```python
from build123d import *

# Parameters (mm, degrees)
SKETCH_1_R          = 45
EXTRUDE_1_DEPTH     = 5
SKETCH_2_W          = 60
SKETCH_2_H          = 60
EXTRUDE_2_DEPTH     = 5
CUT_EXTRUDE_1_DEPTH = 10
CUT_EXTRUDE_START   = -50
CUT_EXTRUDE_2_DEPTH = 10
CUT_EXTRUDE_3_DEPTH = 17
CUT_EXTRUDE_START_2 = -43
CUT_EXTRUDE_4_DEPTH = 17
CUT_EXTRUDE_5_REACH = 89.607
CHAMFER_1_SIZE      = 5
SKETCH_6_R          = 17.5
CUT_EXTRUDE_6_DEPTH = 3
SKETCH_7_R          = 15
CUT_EXTRUDE_7_DEPTH = 65.02343321
SKETCH_8_R          = 45
CUT_EXTRUDE_9_DEPTH = 10


with BuildPart() as part:
    # 草图1 → 凸台-拉伸1 (new body)
    with BuildSketch(Plane.XY):
        Circle(SKETCH_1_R)
    extrude(amount=-EXTRUDE_1_DEPTH)

    # 草图2 → 凸台-拉伸2 (add)
    with BuildSketch(Plane.XY):
        Rectangle(SKETCH_2_W, SKETCH_2_H)
    extrude(amount=EXTRUDE_2_DEPTH)

    # 草图3 → 切除-拉伸1 (cut)
    with BuildSketch(Plane.XZ.offset(30)):
        with BuildLine():
            Line((-1.5, 5), (1.5, 5))
            Line((1.5, 5), (1.5, 4.322875656))
            ThreePointArc((1.5, 4.322875656), (1.780042303, 3.911838473), (1.95, 3.444409721))
            Line((1.95, 3.444409721), (1.95, 2.2))
            Line((1.95, 2.2), (-1.95, 2.2))
            Line((-1.95, 2.2), (-1.95, 3.444409721))
            ThreePointArc((-1.95, 3.444409721), (-1.780042303, 3.911838473), (-1.5, 4.322875656))
            Line((-1.5, 4.322875656), (-1.5, 5))
        make_face()
        with BuildLine():
            Line((6, 5), (6, 4.322875656))
            ThreePointArc((6, 4.322875656), (5.719957697, 3.911838473), (5.55, 3.444409721))
            Line((5.55, 3.444409721), (5.55, 2.2))
            Line((5.55, 2.2), (9.45, 2.2))
            Line((9.45, 2.2), (9.45, 3.444409721))
            ThreePointArc((9.45, 3.444409721), (9.280042303, 3.911838473), (9, 4.322875656))
            Line((9, 4.322875656), (9, 5))
            Line((9, 5), (6, 5))
        make_face()
        with BuildLine():
            Line((-9, 5), (-9, 4.322875656))
            ThreePointArc((-9, 4.322875656), (-9.280042303, 3.911838473), (-9.45, 3.444409721))
            Line((-9.45, 3.444409721), (-9.45, 2.2))
            Line((-9.45, 2.2), (-5.55, 2.2))
            Line((-5.55, 2.2), (-5.55, 3.444409721))
            ThreePointArc((-5.55, 3.444409721), (-5.719957697, 3.911838473), (-6, 4.322875656))
            Line((-6, 4.322875656), (-6, 5))
            Line((-6, 5), (-9, 5))
        make_face()
    extrude(amount=-CUT_EXTRUDE_1_DEPTH, mode=Mode.SUBTRACT)

    # 草图3<2> → 切除-拉伸2 (cut)
    with BuildSketch(Plane.XZ.offset(30).offset(CUT_EXTRUDE_START)):
        with BuildLine():
            Line((-1.5, 5), (1.5, 5))
            Line((1.5, 5), (1.5, 4.322875656))
            ThreePointArc((1.5, 4.322875656), (1.780042303, 3.911838473), (1.95, 3.444409721))
            Line((1.95, 3.444409721), (1.95, 2.2))
            Line((1.95, 2.2), (-1.95, 2.2))
            Line((-1.95, 2.2), (-1.95, 3.444409721))
            ThreePointArc((-1.95, 3.444409721), (-1.780042303, 3.911838473), (-1.5, 4.322875656))
            Line((-1.5, 4.322875656), (-1.5, 5))
        make_face()
        with BuildLine():
            Line((6, 5), (6, 4.322875656))
            ThreePointArc((6, 4.322875656), (5.719957697, 3.911838473), (5.55, 3.444409721))
            Line((5.55, 3.444409721), (5.55, 2.2))
            Line((5.55, 2.2), (9.45, 2.2))
            Line((9.45, 2.2), (9.45, 3.444409721))
            ThreePointArc((9.45, 3.444409721), (9.280042303, 3.911838473), (9, 4.322875656))
            Line((9, 4.322875656), (9, 5))
            Line((9, 5), (6, 5))
        make_face()
        with BuildLine():
            Line((-9, 5), (-9, 4.322875656))
            ThreePointArc((-9, 4.322875656), (-9.280042303, 3.911838473), (-9.45, 3.444409721))
            Line((-9.45, 3.444409721), (-9.45, 2.2))
            Line((-9.45, 2.2), (-5.55, 2.2))
            Line((-5.55, 2.2), (-5.55, 3.444409721))
            ThreePointArc((-5.55, 3.444409721), (-5.719957697, 3.911838473), (-6, 4.322875656))
            Line((-6, 4.322875656), (-6, 5))
            Line((-6, 5), (-9, 5))
        make_face()
    extrude(amount=-CUT_EXTRUDE_2_DEPTH, mode=Mode.SUBTRACT)

    # 草图4 → 切除-拉伸3 (cut)
    with BuildSketch(Plane.XZ.offset(30)):
        with BuildLine():
            Line((-16.5, 5), (-13.5, 5))
            Line((-13.5, 5), (-13.5, 4.322875656))
            ThreePointArc((-13.5, 4.322875656), (-13.219957697, 3.911838473), (-13.05, 3.444409721))
            Line((-13.05, 3.444409721), (-13.05, 2.2))
            Line((-13.05, 2.2), (-16.95, 2.2))
            Line((-16.95, 2.2), (-16.95, 3.444409721))
            ThreePointArc((-16.95, 3.444409721), (-16.780042303, 3.911838473), (-16.5, 4.322875656))
            Line((-16.5, 4.322875656), (-16.5, 5))
        make_face()
        with BuildLine():
            Line((13.5, 5), (16.5, 5))
            Line((16.5, 5), (16.5, 4.322875656))
            ThreePointArc((16.5, 4.322875656), (16.780042303, 3.911838473), (16.95, 3.444409721))
            Line((16.95, 3.444409721), (16.95, 2.2))
            Line((16.95, 2.2), (13.05, 2.2))
            Line((13.05, 2.2), (13.05, 3.444409721))
            ThreePointArc((13.05, 3.444409721), (13.219957697, 3.911838473), (13.5, 4.322875656))
            Line((13.5, 4.322875656), (13.5, 5))
        make_face()
    extrude(amount=-CUT_EXTRUDE_3_DEPTH, mode=Mode.SUBTRACT)

    # 草图4<2> → 切除-拉伸4 (cut)
    with BuildSketch(Plane.XZ.offset(30).offset(CUT_EXTRUDE_START_2)):
        with BuildLine():
            Line((-16.5, 5), (-13.5, 5))
            Line((-13.5, 5), (-13.5, 4.322875656))
            ThreePointArc((-13.5, 4.322875656), (-13.219957697, 3.911838473), (-13.05, 3.444409721))
            Line((-13.05, 3.444409721), (-13.05, 2.2))
            Line((-13.05, 2.2), (-16.95, 2.2))
            Line((-16.95, 2.2), (-16.95, 3.444409721))
            ThreePointArc((-16.95, 3.444409721), (-16.780042303, 3.911838473), (-16.5, 4.322875656))
            Line((-16.5, 4.322875656), (-16.5, 5))
        make_face()
        with BuildLine():
            Line((13.5, 5), (16.5, 5))
            Line((16.5, 5), (16.5, 4.322875656))
            ThreePointArc((16.5, 4.322875656), (16.780042303, 3.911838473), (16.95, 3.444409721))
            Line((16.95, 3.444409721), (16.95, 2.2))
            Line((16.95, 2.2), (13.05, 2.2))
            Line((13.05, 2.2), (13.05, 3.444409721))
            ThreePointArc((13.05, 3.444409721), (13.219957697, 3.911838473), (13.5, 4.322875656))
            Line((13.5, 4.322875656), (13.5, 5))
        make_face()
    extrude(amount=-CUT_EXTRUDE_4_DEPTH, mode=Mode.SUBTRACT)

    # 草图5 → 切除-拉伸5 (cut, up to next)
    with BuildSketch(Plane.XZ.offset(30), mode=Mode.PRIVATE) as cut_extrude_5_sk1:
        with BuildLine():
            Line((-21, 5), (-21, 4.322875656))
            ThreePointArc((-21, 4.322875656), (-20.719957697, 3.911838473), (-20.55, 3.444409721))
            Line((-20.55, 3.444409721), (-20.55, 2.2))
            Line((-20.55, 2.2), (-24.45, 2.2))
            Line((-24.45, 2.2), (-24.45, 3.444409721))
            ThreePointArc((-24.45, 3.444409721), (-24.280042303, 3.911838473), (-24, 4.322875656))
            Line((-24, 4.322875656), (-24, 5))
            Line((-24, 5), (-21, 5))
        make_face()
    cut_extrude_5_tool1 = extrude(cut_extrude_5_sk1.sketch, amount=-CUT_EXTRUDE_5_REACH, mode=Mode.PRIVATE) & part.part
    # 草图5 → 切除-拉伸5 (cut, up to next)
    with BuildSketch(Plane.XZ.offset(30), mode=Mode.PRIVATE) as cut_extrude_5_sk2:
        with BuildLine():
            Line((24, 5), (24, 4.322875656))
            ThreePointArc((24, 4.322875656), (24.280042303, 3.911838473), (24.45, 3.444409721))
            Line((24.45, 3.444409721), (24.45, 2.2))
            Line((24.45, 2.2), (20.55, 2.2))
            Line((20.55, 2.2), (20.55, 3.444409721))
            ThreePointArc((20.55, 3.444409721), (20.719957697, 3.911838473), (21, 4.322875656))
            Line((21, 4.322875656), (21, 5))
            Line((21, 5), (24, 5))
        make_face()
    cut_extrude_5_tool2 = extrude(cut_extrude_5_sk2.sketch, amount=-CUT_EXTRUDE_5_REACH, mode=Mode.PRIVATE) & part.part
    add(cut_extrude_5_tool1.solids().sort_by_distance((-22.5, -30, 3.520698))[0], mode=Mode.SUBTRACT)
    add(cut_extrude_5_tool2.solids().sort_by_distance((22.5, -30, 3.520698))[0], mode=Mode.SUBTRACT)

    # 倒角1
    chamfer_1_edges = [part.edges().sort_by_distance(p)[0] for p in [
        (-30, 30, 2.5),
        (-30, -30, 2.5),
        (30, -30, 2.5),
        (30, 30, 2.5),
    ]]
    chamfer(chamfer_1_edges, length=CHAMFER_1_SIZE)

    # 草图6 → 切除-拉伸6 (cut)
    with BuildSketch(Plane.XY.offset(5)):
        Circle(SKETCH_6_R)
    extrude(amount=-CUT_EXTRUDE_6_DEPTH, mode=Mode.SUBTRACT)

    # 草图7 → 切除-拉伸7 (cut, through all)
    with BuildSketch(Plane.XY.offset(2)):
        Circle(SKETCH_7_R)
    extrude(amount=-CUT_EXTRUDE_7_DEPTH, mode=Mode.SUBTRACT)

    # 草图8 → 切除-拉伸9 (cut)
    with BuildSketch(Plane.XY):
        Circle(SKETCH_8_R)
    extrude(amount=-CUT_EXTRUDE_9_DEPTH, mode=Mode.SUBTRACT)


solid = part.part
```
For this review, take the finished solid that the model builds, in its own axes (mm). A direction names the side the tool comes from. Round coordinates to 2 decimals unless told otherwise and drop trailing zeros. Write each loop counter-clockwise with the first axis right and the second up, starting at its lowest first coordinate (ties: lowest second). Pieces come first, ordered by that corner, then holes. Notation, with made-up numbers: (74, 49.5) - (133, 49.5) arc R21 cw to (133, 57.5) - close; hole circle Ø8 at (74.25, -35.75). An arc over 180 degrees is marked (long way). Answer as CSV lines item,"result". Start each with the question number.
(1) Add section D-D, the plane x = 11. State the section outline as (y, z) points, plus the area to 3 significant figures.
(2) Add section B-B, the plane y = 0. State the section outline as (x, z) points, plus the area to 3 significant figures.
(3) Machinability: for faces 1 (the cylindrical face through (-13.887, -10.648, 3.521)), 2 (the flat face through (0, -25, 2.2)), 3 (the flat face through (23, 0, 2.2)), 4 (the flat face through (-8, 20, 4)), which of the approach directions +Z, -Z, +X, -X, +Y, -Y give a long, thin tool a straight path to every point of the face, cutting with its end or side? Answer none if there is none.
(4) Add section C-C, the plane z = 1.05. State the section outline as (x, y) points.
(5) Mouldability with a two-part tool opening along Y and no side actions: class faces 5 (the flat face through (15, -22, 2.2)), 6 (the cylindrical face through (-14.985, 0.66, 1.014)), 7 (the flat face through (-8, -20, 4)) as +Y half, -Y half, draft (parallel to the pull), parting line (faces both ways), or undercut.
(6) For line 1 (Y direction, x = 0, z = 1.15); line 2 (Y direction, x = 0, z = 3.75); line 3 (X direction, y = -5, z = 1.4), list the stretches that pass through material, from the lowest coordinate up.
(7) For pin 1 (0.8 mm diameter, centred on x = 14.5, z = 3.5, fed in from +Y); pin 2 (0.8 mm diameter, centred on x = -8, z = 4, fed in from -Y); pin 3 (0.8 mm diameter, centred on x = 15.5, z = 4, fed in from -Y), all flat-tipped, find the tip position at first contact; note any pin that passes through.
(8) Add section A-A, the plane x = 0. State the section outline as (y, z) points, plus the area to 3 significant figures.
From the geometry:
1,outline,"(-30, 0) - (-10.2, 0) - (-10.2, 2) - (-13.61, 2) - (-13.61, 5) - (-30, 5) - close; (10.2, 0) - (30, 0) - (30, 5) - (13.61, 5) - (13.61, 2) - (10.2, 2) - close"
1,area,"178 mm²"
2,outline,"(-30, 0) - (-15, 0) - (-15, 2) - (-17.5, 2) - (-17.5, 5) - (-21, 5) - (-21, 4.32) arc R2 cw to (-20.55, 3.44) - (-20.55, 2.2) - (-24.45, 2.2) - (-24.45, 3.44) arc R2 cw to (-24, 4.32) - (-24, 5) - (-30, 5) - close; (15, 0) - (30, 0) - (30, 5) - (24, 5) - (24, 4.32) arc R2 cw to (24.45, 3.44) - (24.45, 2.2) - (20.55, 2.2) - (20.55, 3.44) arc R2 cw to (21, 4.32) - (21, 5) - (17.5, 5) - (17.5, 2) - (15, 2) - close"
2,area,"115 mm²"
3,face 1,"+Z"
3,face 2,"-Y"
3,face 3,"+Y, -Y"
3,face 4,"+Y"
4,outline,"(-30, -25) - (-25, -30) - (25, -30) - (30, -25) - (30, 25) - (25, 30) - (-25, 30) - (-30, 25) - close; hole circle Ø30 at (0, 0)"
5,face 5,"draft"
5,face 6,"undercut"
5,face 7,"-Y half"
6,line 1,"y = -30 to -15, 15 to 30"
6,line 2,"y = -20 to -17.5, 17.5 to 20"
6,line 3,"x = -30 to -14.14, 14.14 to 30"
7,pin 1,"stops at y = 13"
7,pin 2,"stops at y = -20"
7,pin 3,"stops at y = -13"
8,outline,"(-30, 0) - (-15, 0) - (-15, 2) - (-17.5, 2) - (-17.5, 5) - (-20, 5) - (-20, 2.2) - (-30, 2.2) - close; (15, 0) - (30, 0) - (30, 2.2) - (20, 2.2) - (20, 5) - (17.5, 5) - (17.5, 2) - (15, 2) - close"
8,area,"79.0 mm²"
